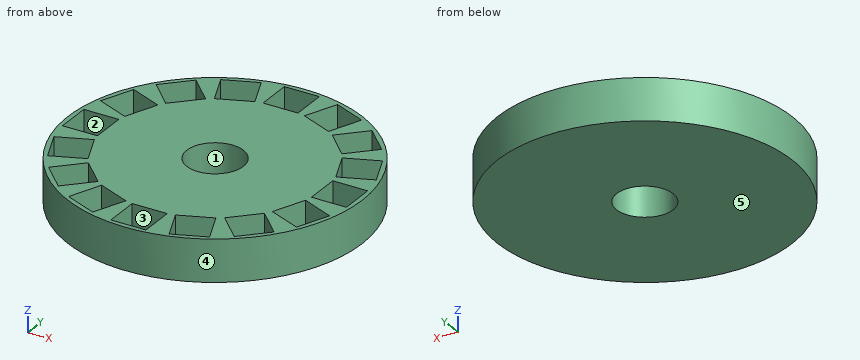
from build123d import *

# Parameters (mm, degrees)
F0_W     = 21
F0_H     = 6
F2_R     = 4.05
F3_DEPTH = 25
F4_W     = 5
F4_H     = 5
F5_DEPTH = 5


# Not quite as in the source:
# - a feature names something its author has since deleted; it is built from what else it names


with BuildPart() as f1:
    # F0 (on Front) → F1 (revolve)
    with BuildSketch(Plane.XZ):
        with Locations((10.5, 3)):
            Rectangle(F0_W, F0_H)
    revolve(axis=Axis((0, 0, 3), (0, 0, -1)))

    # F2 (on Top) → F3 (cut)
    with BuildSketch(Plane.XY):
        Circle(F2_R)
    extrude(amount=F3_DEPTH, mode=Mode.SUBTRACT)

    # F4 (on face) → F5 (cut)
    with BuildSketch(Plane.XY.offset(6)):
        with Locations((0, 17.8)):
            Rectangle(F4_W, F4_H)
        Polygon((3.5453576839, 15.0920654283), (8.1647553465, 13.1786482665), (10.0781725083, 17.7980459291), (5.4587748457, 19.7114630909), align=None)
        Polygon((9.0509667992, 12.5865007051), (12.5865007051, 9.0509667992), (16.1220346111, 12.5865007051), (12.5865007051, 16.1220346111), align=None)
        Polygon((13.1786482665, 8.1647553465), (15.0920654283, 3.5453576839), (19.7114630909, 5.4587748457), (17.7980459291, 10.0781725083), align=None)
        with Locations((17.8, 0)):
            Rectangle(F4_W, F4_H)
        Polygon((15.0920654283, -3.5453576839), (13.1786482665, -8.1647553465), (17.7980459291, -10.0781725083), (19.7114630909, -5.4587748457), align=None)
        Polygon((12.5865007051, -9.0509667992), (9.0509667992, -12.5865007051), (12.5865007051, -16.1220346111), (16.1220346111, -12.5865007051), align=None)
        Polygon((8.1647553465, -13.1786482665), (3.5453576839, -15.0920654283), (5.4587748457, -19.7114630909), (10.0781725083, -17.7980459291), align=None)
        with Locations((0, -17.8)):
            Rectangle(F4_W, F4_H)
        Polygon((-3.5453576839, -15.0920654283), (-8.1647553465, -13.1786482665), (-10.0781725083, -17.7980459291), (-5.4587748457, -19.7114630909), align=None)
        Polygon((-9.0509667992, -12.5865007051), (-12.5865007051, -9.0509667992), (-16.1220346111, -12.5865007051), (-12.5865007051, -16.1220346111), align=None)
        Polygon((-13.1786482665, -8.1647553465), (-15.0920654283, -3.5453576839), (-19.7114630909, -5.4587748457), (-17.7980459291, -10.0781725083), align=None)
        with Locations((-17.8, 0)):
            Rectangle(F4_W, F4_H)
        Polygon((-15.0920654283, 3.5453576839), (-13.1786482665, 8.1647553465), (-17.7980459291, 10.0781725083), (-19.7114630909, 5.4587748457), align=None)
        Polygon((-12.5865007051, 9.0509667992), (-9.0509667992, 12.5865007051), (-12.5865007051, 16.1220346111), (-16.1220346111, 12.5865007051), align=None)
        Polygon((-8.1647553465, 13.1786482665), (-3.5453576839, 15.0920654283), (-5.4587748457, 19.7114630909), (-10.0781725083, 17.7980459291), align=None)
    extrude(amount=-F5_DEPTH, mode=Mode.SUBTRACT)


solid = f1.part
Source: CAD feature listing. Evaluate the final solid. Frame: model axes, mm. Face numbers are marked on the shaded views. A direction names the side the tool comes from. Round coordinates to 2 decimals unless told otherwise and drop trailing zeros. Loops run counter-clockwise (first coordinate to the right, second up) from the corner with the lowest first, then second, coordinate; pieces in that order, holes last. Notation, with made-up numbers: M 8.5,49.25 L 51.5,49.25 A12 cw 51.5,55.25 Z; hole C 31,61.25 d3. An arc over 180 degrees is marked long. Return JSON: item names as keys, results as strings. Group by question number.
1. Mould query, pull axis X, two halves, no side actions, for the marked faces 3, 4 and 5. Classes: released by +X, released by -X, zero draft, split by the parting line, or undercut.
2. Reachability of the marked faces 1 and 2 from +Z, -Z, +X, -X, +Y, -Y: full face, straight path, thin tool, end or side. Return the list, or none.
3. Material intervals for line 1 along X through (y, z) = (0, 2.5); line 2 along X through (y, z) = (-8.5, 4.4), sorted ascending. Write a range as from..to.
4. Section query A-A on x = 0. Output: boundary loops of the cut face in (y, z), and give its area (3 significant figures).
5. Section query C-C on z = 0.5. Output: boundary loops of the cut face in (x, y).
6. Pin query (flat end, axial travel): pin 1 (2.5 mm diameter, centred on x = -0.5, y = -18.5, fed in from +Z); pin 2 (3 mm diameter, centred on y = -14.5, z = 2, fed in from -X); pin 3 (1.5 mm diameter, centred on x = -14, z = 4.5, fed in from +Y). Return the tip coordinate at first contact, or that it passes through.
7. Section query D-D on x = -7. Output: boundary loops of the cut face in (y, z), and give its area (3 significant figures).
Checks:
{
 "1": {"face 3": "undercut", "face 4": "split by the parting line", "face 5": "zero draft"},
 "2": {"face 1": "+Z, -Z", "face 2": "+Z"},
 "3": {"line 1": "x = -21..-20.3, -15.3..-4.05, 4.05..15.3, 20.3..21", "line 2": "x = -19.2..-18.45, -13.99..13.99, 18.45..19.2"},
 "4": {"outline": "M -21,0 L -4.05,0 L -4.05,6 L -15.3,6 L -15.3,1 L -20.3,1 L -20.3,6 L -21,6 Z; M 4.05,0 L 21,0 L 21,6 L 20.3,6 L 20.3,1 L 15.3,1 L 15.3,6 L 4.05,6 Z", "area": "153 mm²"},
 "5": {"outline": "C 0,0 d42; hole C 0,0 d8.1"},
 "6": {"pin 1": "stops at z = 1", "pin 2": "stops at x = -16.49", "pin 3": "stops at y = 16.29"},
 "7": {"outline": "M -19.8,0 L 19.8,0 L 19.8,6 L 19.07,6 L 19.07,1 L 13.66,1 L 13.66,6 L -13.66,6 L -13.66,1 L -19.07,1 L -19.07,6 L -19.8,6 Z", "area": "183 mm²"}
}
